Print and shaded views of the part. All mm, measured from the part's lowest x, y and z. A direction names the side the tool comes from. Coordinates: 2 decimals unless noted, no trailing zeros. Loops run counter-clockwise (first coordinate to the right, second up) from the corner with the lowest first, then second, coordinate; pieces in that order, holes last. Notation, with made-up numbers: M 13.25,32.25 L 70.25,32.25 A19 ccw 70.25,51.25 Z; hole C 9.25,54.5 d8. An arc over 180 degrees is marked long. Answer as a JSON object with one key per item and string values. Group by question number.
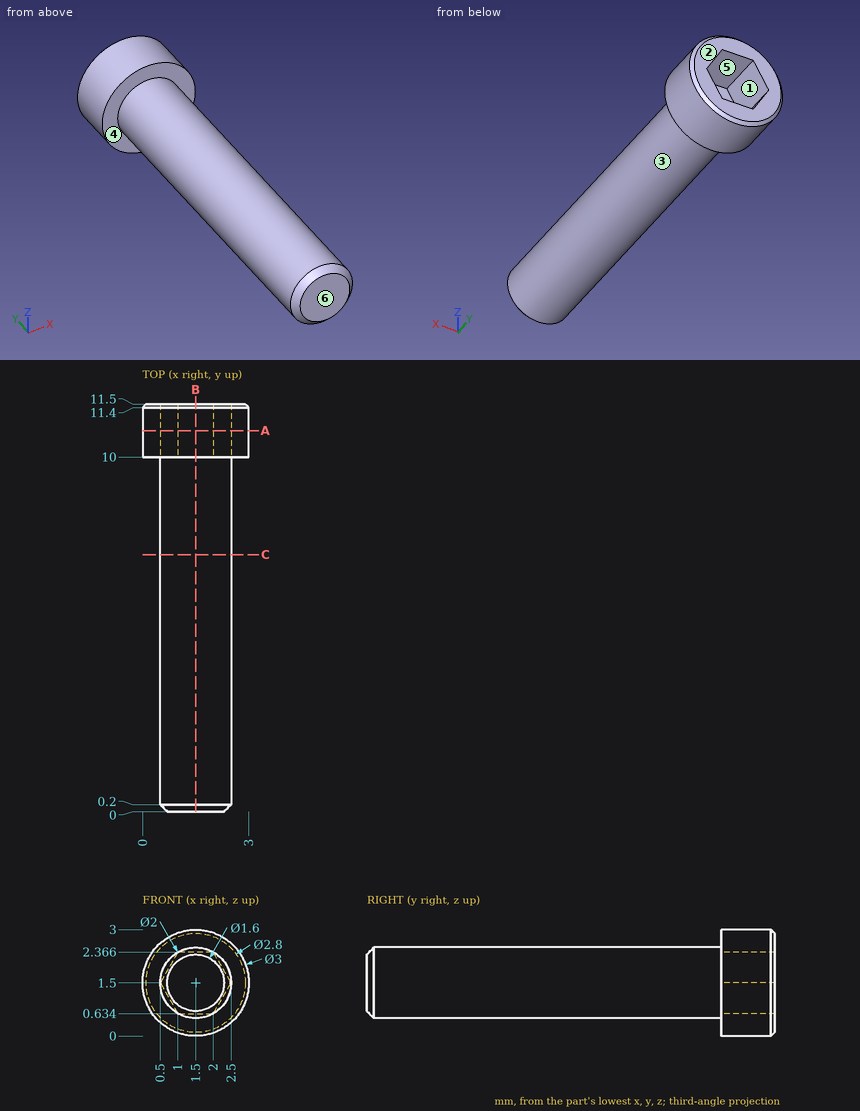
Item 1: Pull direction Z, two halves, no side cores. Call the marked faces 1, 2 and 3: released by +Z, released by -Z, zero draft, split by the parting line, or undercut.
Item 2: Pin check, flat tip, straight feed: pin 1 (0.5 mm diameter, centred on x = 1, z = 1.5, fed in from +Y). Stop position of the tip, or through.
Item 3: Drill centre lines: L1, parallel to Y at x = 0.4, z = 1.4; L2, parallel to X at y = 8, z = 1.6; L3, parallel to X at y = 4.5, z = 2.1. Where is each one in solid material? Low to high. Write a range as from..to.
Item 4: Slice it at B-B, the plane x = 1.5. Write the cut outline in (y, z), then the cut area to 3 significant figures.
Item 5: Slice it at A-A, the plane y = 10.75. Write the cut outline in (x, z), then the cut area to 3 significant figures.
Item 6: Tool access for the marked faces 4, 5 and 6: list every direction of +Z, -Z, +X, -X, +Y, -Y with a clear straight run to the whole face (end or side of a thin tool).
Item 7: Slice it at C-C, the plane y = 7.25. Write the cut outline in (x, z).
Computed:
{
 "1": {"face 1": "undercut", "face 2": "zero draft", "face 3": "split by the parting line"},
 "2": {"pin 1": "y = 10"},
 "3": {"L1": "10..11.5", "L2": "0.51..2.49", "L3": "0.7..2.3"},
 "4": {"outline": "M 0,0.7 L 0.2,0.5 L 10,0.5 L 10,0 L 11.4,0 L 11.5,0.1 L 11.5,0.63 L 10,0.63 L 10,2.37 L 11.5,2.37 L 11.5,2.9 L 11.4,3 L 10,3 L 10,2.5 L 0.2,2.5 L 0,2.3 Z", "area": "21.9 mm2"},
 "5": {"outline": "C 1.5,1.5 d3; hole M 0.5,1.5 L 1,0.63 L 2,0.63 L 2.5,1.5 L 2,2.37 L 1,2.37 Z", "area": "4.47 mm2"},
 "6": {"face 4": "-Y", "face 5": "+Y", "face 6": "+Z, -Z, +X, -X, -Y"},
 "7": {"outline": "C 1.5,1.5 d2"}
}
